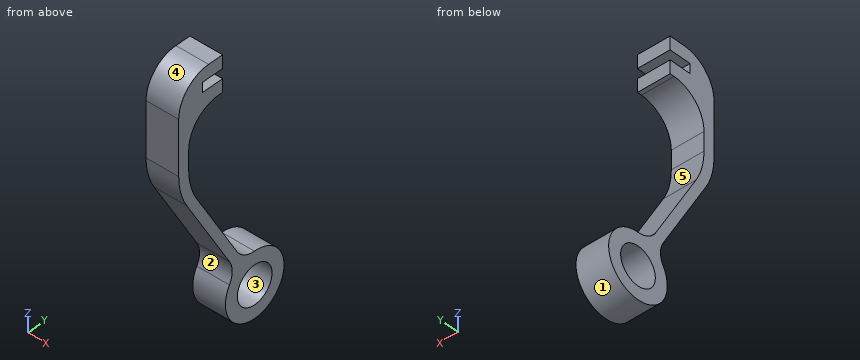
```python
from build123d import *

# Parameters (mm, degrees)
F0_R     = 4.35
F1_DEPTH = 7.5
F2_R     = 7.5


with BuildPart() as f1:
    # F0 (on Right) → F1 (new body)
    with BuildSketch(Plane.YZ):
        with BuildLine():
            Line((0, 15.8), (0, 18.8))
            Line((0, 18.8), (-5, 18.8))
            Line((-5, 18.8), (-5, 21))
            Line((-5, 21), (0, 21))
            Line((0, 21), (0, 24))
            Line((0, 24), (-11, 24))
            Line((-11, 24), (-11, 4.019238))
            ThreePointArc((-11, 4.019238), (-10.488887, 0.136952), (-8.990381, -3.480762))
            Line((-8.990381, -3.480762), (1.750865, -22.085146))
            ThreePointArc((1.750865, -22.085146), (2.420692, -24.606707), (1.729144, -27.122397))
            ThreePointArc((1.729144, -27.122397), (11.7375, -37.217442), (7.999113, -23.502428))
            ThreePointArc((7.999113, -23.502428), (5.474687, -22.843481), (3.625865, -21.002614))
            Line((3.625865, -21.002614), (-6.490381, -3.480762))
            ThreePointArc((-6.490381, -3.480762), (-7.988887, 0.136952), (-8.5, 4.019238))
            Line((-8.5, 4.019238), (-8.5, 15.8))
            Line((-8.5, 15.8), (0, 15.8))
        make_face()
        with Locations((8.0625, -30.852155)):
            Circle(F0_R, mode=Mode.SUBTRACT)
    extrude(amount=F1_DEPTH)

    # F2
    f2_edges = [f1.edges().sort_by_distance(p)[0] for p in [
        (3.75, -11, 24),
        (3.75, -8.5, 15.8),
    ]]
    fillet(f2_edges, radius=F2_R)


solid = f1.part
```
Could you check a few things on this model? Use its own coordinates, in mm. Face numbers are marked on the shaded views. A direction names the side the tool comes from. Coordinates: 2 decimals unless noted, no trailing zeros. Write each loop counter-clockwise with the first axis right and the second up, starting at its lowest first coordinate (ties: lowest second). Pieces come first, ordered by that corner, then holes. Notation, with made-up numbers: (-19, 62) - (18, 62) arc R18 ccw to (18, 97) - close; hole circle Ø11 at (83, 11.5). An arc over 180 degrees is marked (long way). Use a Markdown table: item, result.
Q1. Imagine slicing it at D-D (z = 1.5). List the corners of the cut face in (x, y) for me, and give its area (4 significant figures).
Geometry check:
| item | result |
|---|---|
| outline | (0, -10.79) - (7.5, -10.79) - (7.5, -8.29) - (0, -8.29) - close |
| area | 18.75 mm2 |
Q2. Please list where these lines run through material, in increasing order: L1, parallel to Z at x = 4.5, y = -1.5; L2, parallel to Z at x = 3, y = -1.75; L3, parallel to Y at x = 5, z = -31.
Geometry check:
| item | result |
|---|---|
| L1 | z = -16.45 to -12.12, 15.78 to 18.8, 21 to 24 |
| L2 | z = -16.02 to -11.69, 15.76 to 18.8, 21 to 24 |
| L3 | y = 0.71 to 3.72, 12.41 to 15.41 |
Q3. Imagine slicing it at C-C (z = -32). List the corners of the cut face in (x, y) for me.
Geometry check:
| item | result |
|---|---|
| outline | (0, 0.8) - (7.5, 0.8) - (7.5, 3.87) - (0, 3.87) - close; (0, 12.26) - (7.5, 12.26) - (7.5, 15.32) - (0, 15.32) - close |
Q4. Imagine slicing it at A-A (y = 10). List the corners of the cut face in (x, z) for me, and give its area (3 significant figures).
Geometry check:
| item | result |
|---|---|
| outline | (0, -37.94) - (7.5, -37.94) - (7.5, -34.75) - (0, -34.75) - close; (0, -26.96) - (7.5, -26.96) - (7.5, -23.76) - (0, -23.76) - close |
| area | 47.9 mm2 |
Q5. Thinking about a two-plate mould opening in Y: for the marked faces 1, 2 and 3, which applies, +Y half, -Y half, draft (parallel to the pull), parting line (faces both ways), or undercut?
Geometry check:
| item | result |
|---|---|
| face 1 | parting line |
| face 2 | -Y half |
| face 3 | undercut |
Q6. I'm going to push flat-ended pins straight in: pin 1 Ø0.7 at (x, z) = (5, 20) entering from +Y; pin 2 Ø1.5 at (x, z) = (3, 18) entering from +Y; pin 3 Ø4 at (y, z) = (2, -28.5) entering from -X; pin 4 Ø1.3 at (x, z) = (5.5, 6.5) entering from +Y. Where does each tip first touch, or does it pass through?
Geometry check:
| item | result |
|---|---|
| pin 1 | stops at y = -5 |
| pin 2 | stops at y = 0 |
| pin 3 | stops at x = 0 |
| pin 4 | stops at y = -8.5 |
Q7. Which directions (+Z, -Z, +X, -X, +Y, -Y) give clear straight access to the entire face, cutting with the end or side of a thin tool? Please do the marked faces 4 and 5.
Geometry check:
| item | result |
|---|---|
| face 4 | +Z, +X, -X, -Y |
| face 5 | +X, -X, +Y |
Q8. Imagine slicing it at B-B (x = 4.25). List the corners of the cut face in (y, z) for me, and give its area (3 significant figures).
Geometry check:
| item | result |
|---|---|
| outline | (-11, 4.02) arc R15 ccw to (-8.99, -3.48) - (1.75, -22.09) arc R5 cw to (1.73, -27.12) arc R7.35 ccw (long way) to (8, -23.5) arc R5 cw to (3.63, -21) - (-6.49, -3.48) arc R15 cw to (-8.5, 4.02) - (-8.5, 8.3) arc R7.5 cw to (-1, 15.8) - (0, 15.8) - (0, 18.8) - (-5, 18.8) - (-5, 21) - (0, 21) - (0, 24) - (-3.5, 24) arc R7.5 ccw to (-11, 16.5) - close; hole circle Ø8.7 at (8.06, -30.85) |
| area | 294 mm2 |
